Here's how the part is built. I have some questions about the finished solid (model axes, mm). A direction names the side the tool comes from. Coordinates: 2 decimals unless noted, no trailing zeros. Loops run counter-clockwise (first coordinate to the right, second up) from the corner with the lowest first, then second, coordinate; pieces in that order, holes last. Notation, with made-up numbers: M 36,66 L 61,66 A9 ccw 61,72 Z; hole C 66.25,84.25 d6. An arc over 180 degrees is marked long. Use one line per item in the form item = value. Start each with the question number.
(1) Imagine slicing it at D-D, the plane y = -58.5. Please give me the cut outline in (x, z).
(2) Imagine slicing it at A-A, the plane y = 4. Please give me the cut outline in (x, z), and give its area (3 significant figures).
(3) On a 3-axis mill with a long thin cutter (end or side, diameter ignored), from which of +Z, -Z, +X, -X, +Y, -Y can I reach the whole of each face in a straight line? I mean faces 4 (the cylindrical face through (-16.1, -10.73, -0.91)), 5 (the flat face through (10.75, -13, 5)), 6 (the flat face through (-42, -118, 9)), 7 (the cylindrical face through (-36.102, -28.382, -0.938)), 8 (the flat face through (-6, 12.35, 4)). Say none if no direction works.
(4) Please list where these lines run through material, in increasing order: L1, parallel to Y at x = -1, z = 1.5; L2, parallel to X at y = -13, z = 2.5; L3, parallel to Y at x = 0, z = -0.9.
(5) Thinking about a two-plate mould opening in X: for faces 1 (the flat face through (2, -118, 9)), 2 (the cylindrical face through (-5.398, -102.758, -0.912)), 3 (the cylindrical face through (-49.24, -114.65, 4.44)), which applies, +X half, -X half, draft (parallel to the pull), parting line (faces both ways), or undercut?
(6) Imagine slicing it at C-C, the plane z = 1.5. State how many separate pieces and enclosed holes the cut face has, and give its area (3 significant figures).
(7) Imagine slicing it at B-B, the plane x = -37. Please give me the cut outline in (y, z).
(8) Will these pins go through, and if not, where does the flat tip stop? P1, Ø1.5, axis at y = -59, z = 2, coming from the +X side; P2, Ø19, axis at x = -8.5, y = -51, coming from the +Z side; P3, Ø3, axis at x = -47.5, z = 5, coming from the +Y side; P4, Ø3, axis at y = -47.5, z = 0.5, coming from the +X side.
```python
from build123d import *

# Parameters (mm, degrees)
F3_W     = 1.85
F3_H     = 9
F1_R     = 2
F5_DEPTH = 1.85
F6_W     = 25.2441216726
F6_H     = 31.736315228
F6_W_2   = 15
F6_H_2   = 17.6660341024
F6_W_3   = 32.0804953698
F6_H_3   = 80.390445888
F6_W_4   = 30.8194325197
F7_DEPTH = 25
F8_R     = 10
F9_SIZE  = 1


with BuildPart() as f4:
    # F4: sweep along a path in F1
    with BuildLine(Plane.XY) as f4_path:
        Line((10.75, 0.5), (10.75, -107.5))
        ThreePointArc((10.75, -107.5), (7.8210678119, -114.5710678119), (0.75, -117.5))
        Line((0.75, -117.5), (-42.25, -117.5))
        ThreePointArc((-42.25, -117.5), (-49.3210678119, -114.5710678119), (-52.25, -107.5))
        Line((-52.25, -107.5), (-52.25, 0.5))
        ThreePointArc((-52.25, 0.5), (-49.3210678119, 7.5710678119), (-42.25, 10.5))
        Line((-42.25, 10.5), (0.75, 10.5))
        ThreePointArc((0.75, 10.5), (7.8210678119, 7.5710678119), (10.75, 0.5))
    # F3 (on line) → F4 (sweep)
    with BuildSketch(Plane.XZ.offset(53.5)):
        with Locations((11.675, 4.5)):
            Rectangle(F3_W, F3_H)
    sweep(path=f4_path.line)

    # F1 (on Top) → F5 (join)
    with BuildSketch(Plane.XY):
        with BuildLine():
            Line((0.75, 12.35), (-42.25, 12.35))
            ThreePointArc((-42.25, 12.35), (-50.6292153571, 8.8792153571), (-54.1, 0.5))
            Line((-54.1, 0.5), (-54.1, -107.5))
            ThreePointArc((-54.1, -107.5), (-50.6292153571, -115.8792153571), (-42.25, -119.35))
            Line((-42.25, -119.35), (0.75, -119.35))
            ThreePointArc((0.75, -119.35), (9.1292153571, -115.8792153571), (12.6, -107.5))
            Line((12.6, -107.5), (12.6, 0.5))
            ThreePointArc((12.6, 0.5), (9.1292153571, 8.8792153571), (0.75, 12.35))
        make_face()
        with BuildLine():
            Line((-42.25, 10.5), (0.75, 10.5))
            ThreePointArc((0.75, 10.5), (7.8210678119, 7.5710678119), (10.75, 0.5))
            Line((10.75, 0.5), (10.75, -107.5))
            ThreePointArc((10.75, -107.5), (7.8210678119, -114.5710678119), (0.75, -117.5))
            Line((0.75, -117.5), (-42.25, -117.5))
            ThreePointArc((-42.25, -117.5), (-49.3210678119, -114.5710678119), (-52.25, -107.5))
            Line((-52.25, -107.5), (-52.25, 0.5))
            ThreePointArc((-52.25, 0.5), (-49.3210678119, 7.5710678119), (-42.25, 10.5))
        make_face(mode=Mode.SUBTRACT)
        with BuildLine():
            ThreePointArc((10.75, 0.5), (7.8210678119, 7.5710678119), (0.75, 10.5))
            Line((0.75, 10.5), (-42.25, 10.5))
            ThreePointArc((-42.25, 10.5), (-49.3210678119, 7.5710678119), (-52.25, 0.5))
            Line((-52.25, 0.5), (-52.25, -107.5))
            ThreePointArc((-52.25, -107.5), (-49.3210678119, -114.5710678119), (-42.25, -117.5))
            Line((-42.25, -117.5), (0.75, -117.5))
            ThreePointArc((0.75, -117.5), (7.8210678119, -114.5710678119), (10.75, -107.5))
            Line((10.75, -107.5), (10.75, 0.5))
        make_face()
        Circle(F1_R, mode=Mode.SUBTRACT)
    extrude(amount=-F5_DEPTH)

    # F6 (on Top) → F7 (cut, symmetric)
    with BuildSketch(Plane.XY):
        with Locations((-25.8720608363, 2.1293233149)):
            Rectangle(F6_W, F6_H)
        with Locations((-20.75, -126.3330170512)):
            Rectangle(F6_W_2, F6_H_2)
        with Locations((-49.2902476849, -65.5702464283)):
            Rectangle(F6_W_3, F6_H_3)
        with Locations((7.1597162599, -65.5702464283)):
            Rectangle(F6_W_4, F6_H_3)
    extrude(amount=F7_DEPTH, both=True, mode=Mode.SUBTRACT)

    # F8
    f8_edges = [f4.edges().sort_by_distance(p)[0] for p in [
        (-33.25, -25.375023, -0.925),
        (-8.25, -25.375023, -0.925),
        (-8.25, -105.765469, -0.925),
        (-33.25, -105.765469, -0.925),
        (-38.494122, -13.738834, -0.925),
        (-13.25, -13.738834, -0.925),
    ]]
    fillet(f8_edges, radius=F8_R)

    # F9
    f9_edges = [f4.edges().sort_by_distance(p)[0] for p in [
        (-54.1, -25.375023, 3.575),
        (12.6, -25.375023, 3.575),
        (-13.25, 12.35, 3.575),
        (-38.494122, 12.35, 3.575),
        (-54.1, -105.765469, 3.575),
        (12.6, -105.765469, 3.575),
    ]]
    chamfer(f9_edges, length=F9_SIZE)


solid = f4.part
```
Answer:
q1.outline = M -33.25,-1.85 L -8.25,-1.85 L -8.25,0 L -33.25,0 Z
q2.outline = M -53.57,-1.85 L -38.49,-1.85 L -38.49,0 L -51.62,0 L -51.62,9 L -53.57,9 Z; M -13.25,-1.85 L 12.07,-1.85 L 12.07,9 L 10.12,9 L 10.12,0 L -13.25,0 Z
q2.area = 110 mm²
q3.face_4 = +Z, -Z, +Y
q3.face_5 = +Z
q3.face_6 = +Z, +X, -X, +Y, -Y
q3.face_7 = +Z, -Z, -X
q3.face_8 = +Z, -Z, +X, -X, +Y
q4.L1 = -119.35 to -117.5, 10.5 to 12.35
q4.L2 = -54.1 to -52.25, 10.75 to 12.6
q4.L3 = -119.35 to -105.61, -25.53 to -2, 2 to 12.35
q5.face_1 = draft
q5.face_2 = +X half
q5.face_3 = undercut
q6.separate_pieces = 4
q6.enclosed_holes = 0
q6.area = 311 mm²
q7.outline = M -119.35,-1.85 L -103.57,-1.85 L -103.57,0 L -117.5,0 L -117.5,9 L -119.35,9 Z; M -27.57,-1.85 L -9,-1.85 L -9,0 L -27.57,0 Z
q8.P1 = through
q8.P2 = 0
q8.P3 = 11.74
q8.P4 = -8.25
